from build123d import *

# Parameters (mm, degrees)
SKETCH1_R           = 1.625
BOSS_EXTRUDE1_DEPTH = 3
SKETCH3_W           = 5
SKETCH3_H           = 40
BOSS_EXTRUDE3_DEPTH = 5


with BuildPart() as part:
    # Sketch1 → Boss-Extrude1 (new body)
    with BuildSketch(Plane.XY):
        Polygon((0, 0), (0, 40), (-7.5, 40), (-7.5, 47.5), (12.5, 47.5), (12.5, 40), (5, 40), (5, 0), align=None)
        with Locations((-3.75, 43.75)):
            Circle(SKETCH1_R, mode=Mode.SUBTRACT)
        with Locations((8.75, 43.75)):
            Circle(SKETCH1_R, mode=Mode.SUBTRACT)
    extrude(amount=BOSS_EXTRUDE1_DEPTH)

    # Sketch3 → Boss-Extrude3 (add)
    with BuildSketch(Plane(origin=(0, 0, 0), x_dir=(-1, 0, 0), z_dir=(0, 0, -1))):
        with Locations((-2.5, 20)):
            Rectangle(SKETCH3_W, SKETCH3_H)
    extrude(amount=BOSS_EXTRUDE3_DEPTH)


solid = part.part
The model under review builds one solid part; all positions refer to its coordinate system, in mm. A direction names the side the tool comes from. Round coordinates to 2 decimals unless told otherwise and drop trailing zeros. Loops run counter-clockwise (first coordinate to the right, second up) from the corner with the lowest first, then second, coordinate; pieces in that order, holes last. Notation, with made-up numbers: (86.25, 68.5) -> (136.25, 68.5) arc R11 cw to (136.25, 83.5) -> close; hole circle Ø11 at (-34, 12.5). An arc over 180 degrees is marked (long way). Write item = value, one per line. Start each with the question number.
Item 1: Take a section at A-A on x = -3.75. Give the boundary of the cut face in (y, z) (3 decimals), plus the area to 4 significant figures.
Item 2: Take a section at C-C on z = 0.5. Give the boundary of the cut face in (x, y) (3 decimals).
Item 3: Mouldability with a two-part tool opening along X and no side actions: class faces 1 (the flat face through (3, 0, -1)), 2 (the cylindrical face through (-4.102, 42.164, 1.479)), 3 (the flat face through (12.5, 44, 1)), 4 (the flat face through (-7.5, 44, 1)) as released by +X, released by -X, zero draft, split by the parting line, or undercut.
Item 4: Insertion check: pin 1 (2.5 mm diameter, centred on x = -2, z = 2, fed in from -Y); pin 2 (4 mm diameter, centred on y = 20, z = -2.5, fed in from -X); pin 3 (3 mm diameter, centred on x = -3.75, y = 43.75, fed in from -Z); pin 4 (3.5 mm diameter, centred on x = 8.75, y = 43.75, fed in from -Z). Each pin has a flat end and moves straight along its axis. Give the tip position at first contact, or say it passes through.
Item 5: To check wall thickness, follow L1, parallel to Y at x = 8.75, z = 1.25 (3 decimals); L2, parallel to X at y = 26.5, z = 1.5; L3, parallel to Z at x = -2.5, y = 45.5. State the ranges of each line that lie inside material, in increasing order.
Item 6: Take a section at D-D on y = 31.5. Give the boundary of the cut face in (x, z).
Item 7: For faces 5 (the flat face through (3, 20, -5)), 6 (the flat face through (0, 20, -1)), 7 (the flat face through (2, 47.5, 1)), 8 (the flat face through (3, 44, 0)), 9 (the flat face through (9, 40, 1)), list the 3-axis set-ups (+Z, -Z, +X, -X, +Y, -Y) from which the entire face can be reached by the end or side of a thin tool; tool diameter is ignored.
Item 8: Take a section at B-B on y = 43.75. Give the boundary of the cut face in (x, z) (3 decimals).
Result:
q1.outline = (40, 0) -> (42.125, 0) -> (42.125, 3) -> (40, 3) -> close; (45.375, 0) -> (47.5, 0) -> (47.5, 3) -> (45.375, 3) -> close
q1.area = 12.75 mm²
q2.outline = (-7.5, 40) -> (0, 40) -> (0, 0) -> (5, 0) -> (5, 40) -> (12.5, 40) -> (12.5, 47.5) -> (-7.5, 47.5) -> close; hole circle Ø3.25 at (-3.75, 43.75); hole circle Ø3.25 at (8.75, 43.75)
q3.face_1 = zero draft
q3.face_2 = undercut
q3.face_3 = released by +X
q3.face_4 = released by -X
q4.pin_1 = 40
q4.pin_2 = 0
q4.pin_3 = through
q4.pin_4 = 0
q5.L1 = 40 to 42.125, 45.375 to 47.5
q5.L2 = 0 to 5
q5.L3 = 0 to 3
q6.outline = (0, -5) -> (5, -5) -> (5, 3) -> (0, 3) -> close
q7.face_5 = -Z, +X, -X, +Y, -Y
q7.face_6 = +Z, -Z, -X, -Y
q7.face_7 = +Z, -Z, +X, -X, +Y
q7.face_8 = -Z, +X, -X, +Y
q7.face_9 = +Z, -Z, +X, -Y
q8.outline = (-7.5, 0) -> (-5.375, 0) -> (-5.375, 3) -> (-7.5, 3) -> close; (-2.125, 0) -> (7.125, 0) -> (7.125, 3) -> (-2.125, 3) -> close; (10.375, 0) -> (12.5, 0) -> (12.5, 3) -> (10.375, 3) -> close
